Verification items for the finished model (mm, model axes). Coordinates: 2 decimals unless noted, no trailing zeros. Order: outer loops, then holes, each group sorted by start corner. A loop starts at its lowest first (then second) coordinate and runs counter-clockwise, first axis right, second up. Notation, with made-up numbers: (-37.75, 76.25) -> (1.25, 76.25) arc R20 cw to (1.25, 108.25) -> close; hole circle Ø2 at (68.5, 48.25). An arc over 180 degrees is marked (long way). Write item = value, one per line. Start each with the question number.
1. Go/stop test with a flat-tipped pin: P1, Ø1, axis at y = -1, z = 7.5, coming from the +X side. Record where the tip stops, or that it passes through.
2. Cross-section at A-A on x = 36. Record the cut outline in (y, z) (3 decimals), plus the area to 3 significant figures.
3. Thickness scan on line 1 along X through (y, z) = (15, 9.5) (3 decimals); line 2 along Y through (x, z) = (67, 7.5); line 3 along X through (y, z) = (-22, 7.25). Record the ranges inside material, lowest first. Write a range as from..to.
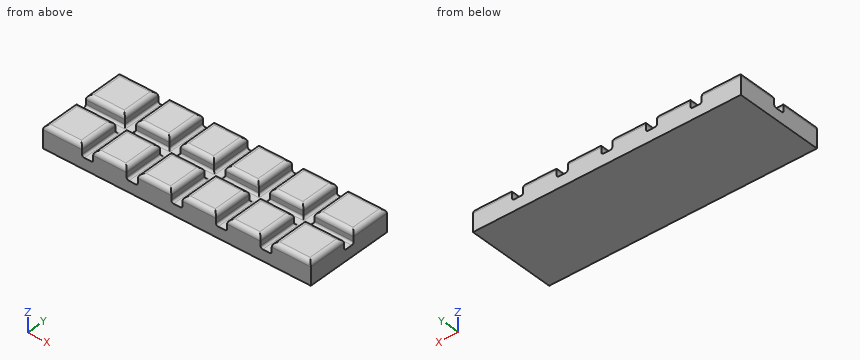
from build123d import *

# Parameters (mm, degrees)
F0_W     = 152.4
F0_H     = 50.8
F1_DEPTH = 12.7
F2_W     = 6.35
F2_H     = 12.7
F3_DEPTH = 152.401
F4_W     = 6.35
F4_H     = 12.7
F5_DEPTH = 50.801
F6_R     = 2.54
F7_R     = 1.27


with BuildPart() as f1:
    # F0 (on Top) → F1 (new body)
    with BuildSketch(Plane.XY):
        Rectangle(F0_W, F0_H)
    extrude(amount=F1_DEPTH)

    # F2 (on face) → F3 (cut, through all)
    with BuildSketch(Plane.YZ.offset(76.2)):
        with Locations((0, 12.7)):
            Rectangle(F2_W, F2_H)
    extrude(amount=-F3_DEPTH, mode=Mode.SUBTRACT)

    # F4 (on face) → F5 (cut, through all)
    with BuildSketch(Plane.XZ.offset(25.4)):
        with Locations((0, 12.7)):
            Rectangle(F4_W, F4_H)
        with Locations((25.4, 12.7)):
            Rectangle(F4_W, F4_H)
        with Locations((50.8, 12.7)):
            Rectangle(F4_W, F4_H)
        with Locations((-25.4, 12.7)):
            Rectangle(F4_W, F4_H)
        with Locations((-50.8, 12.7)):
            Rectangle(F4_W, F4_H)
    extrude(amount=-F5_DEPTH, mode=Mode.SUBTRACT)

    # F6
    f6_edges = [f1.edges().sort_by_distance(p)[0] for p in [
        (-65.0875, -25.4, 12.7),
        (-76.2, -14.2875, 12.7),
        (-65.0875, -3.175, 12.7),
        (-53.975, -14.2875, 12.7),
        (-38.1, -25.4, 12.7),
        (-47.625, -14.2875, 12.7),
        (-38.1, -3.175, 12.7),
        (-28.575, -14.2875, 12.7),
        (-12.7, -25.4, 12.7),
        (-22.225, -14.2875, 12.7),
        (-12.7, -3.175, 12.7),
        (-3.175, -14.2875, 12.7),
        (12.7, -25.4, 12.7),
        (3.175, -14.2875, 12.7),
        (12.7, -3.175, 12.7),
        (22.225, -14.2875, 12.7),
        (38.1, -25.4, 12.7),
        (28.575, -14.2875, 12.7),
        (38.1, -3.175, 12.7),
        (47.625, -14.2875, 12.7),
        (65.0875, -25.4, 12.7),
        (53.975, -14.2875, 12.7),
        (65.0875, -3.175, 12.7),
        (76.2, -14.2875, 12.7),
        (65.0875, 3.175, 12.7),
        (53.975, 14.2875, 12.7),
        (65.0875, 25.4, 12.7),
        (76.2, 14.2875, 12.7),
        (38.1, 3.175, 12.7),
        (28.575, 14.2875, 12.7),
        (38.1, 25.4, 12.7),
        (47.625, 14.2875, 12.7),
        (12.7, 3.175, 12.7),
        (3.175, 14.2875, 12.7),
        (12.7, 25.4, 12.7),
        (22.225, 14.2875, 12.7),
        (-38.1, 3.175, 12.7),
        (-47.625, 14.2875, 12.7),
        (-38.1, 25.4, 12.7),
        (-28.575, 14.2875, 12.7),
        (-12.7, 3.175, 12.7),
        (-22.225, 14.2875, 12.7),
        (-12.7, 25.4, 12.7),
        (-3.175, 14.2875, 12.7),
        (-65.0875, 3.175, 12.7),
        (-76.2, 14.2875, 12.7),
        (-65.0875, 25.4, 12.7),
        (-53.975, 14.2875, 12.7),
    ]]
    fillet(f6_edges, radius=F6_R)

    # F7
    f7_edges = [f1.edges().sort_by_distance(p)[0] for p in [
        (-47.625, 14.2875, 6.35),
        (-53.975, 14.2875, 6.35),
        (-53.975, -14.2875, 6.35),
        (-47.625, -14.2875, 6.35),
        (-22.225, -14.2875, 6.35),
        (-28.575, -14.2875, 6.35),
        (-28.575, 14.2875, 6.35),
        (-22.225, 14.2875, 6.35),
        (3.175, -14.2875, 6.35),
        (3.175, 14.2875, 6.35),
        (-3.175, 14.2875, 6.35),
        (-3.175, -14.2875, 6.35),
        (22.225, 14.2875, 6.35),
        (22.225, -14.2875, 6.35),
        (28.575, -14.2875, 6.35),
        (28.575, 14.2875, 6.35),
        (47.625, 14.2875, 6.35),
        (47.625, -14.2875, 6.35),
        (53.975, 14.2875, 6.35),
        (53.975, -14.2875, 6.35),
        (65.0875, -3.175, 6.35),
        (38.1, -3.175, 6.35),
        (12.7, -3.175, 6.35),
        (-12.7, -3.175, 6.35),
        (-38.1, -3.175, 6.35),
        (-65.0875, -3.175, 6.35),
        (-65.0875, 3.175, 6.35),
        (-12.7, 3.175, 6.35),
        (-38.1, 3.175, 6.35),
        (12.7, 3.175, 6.35),
        (38.1, 3.175, 6.35),
        (65.0875, 3.175, 6.35),
    ]]
    fillet(f7_edges, radius=F7_R)


solid = f1.part
Worked out:
q1.P1 = through
q2.outline = (-25.4, 0) -> (25.4, 0) -> (25.4, 10.16) arc R2.54 ccw to (22.86, 12.7) -> (5.715, 12.7) arc R2.54 ccw to (3.175, 10.16) -> (3.175, 7.62) arc R1.27 cw to (1.905, 6.35) -> (-1.905, 6.35) arc R1.27 cw to (-3.175, 7.62) -> (-3.175, 10.16) arc R2.54 ccw to (-5.715, 12.7) -> (-22.86, 12.7) arc R2.54 ccw to (-25.4, 10.16) -> close
q2.area = 600 mm²
q3.line_1 = -76.2..-53.975, -47.625..-28.575, -22.225..-3.175, 3.175..22.225, 28.575..47.625, 53.975..76.2
q3.line_2 = -25.4..-3.17, 3.17..25.4
q3.line_3 = -76.2..-53.92, -47.68..-28.52, -22.28..-3.12, 3.12..22.28, 28.52..47.68, 53.92..76.2
